The model under review builds one solid part; all positions refer to its coordinate system, in mm. A direction names the side the tool comes from. Coordinates: 2 decimals unless noted, no trailing zeros. Order: outer loops, then holes, each group sorted by start corner. A loop starts at its lowest first (then second) coordinate and runs counter-clockwise, first axis right, second up. Notation, with made-up numbers: M 56.5,84.25 L 68.5,84.25 A21 cw 68.5,101.25 Z; hole C 47,71 d6. An arc over 180 degrees is marked long. One line per item, written item: value.
```python
from build123d import *

# Parameters (mm, degrees)
F0_W         = 5
F0_H         = 5
F1_DEPTH     = 5
F2_DEPTH     = 15
F2_TAPER     = 5
F4_DEPTH     = 2.5
F5_T4_DEPTH  = 8.4
F5_T9_DEPTH  = 8.4
F5_T14_DEPTH = 8.4
F5_T19_DEPTH = 8.4
F5_T24_DEPTH = 8.4
F5_T29_DEPTH = 8.4
F5_T34_DEPTH = 8.4
F5_T39_DEPTH = 8.4
F6_T1_DEPTH  = 65.9153400942
F6_T6_DEPTH  = 63.5246599058
F6_T12_DEPTH = 63.5246599058


# Not quite as in the source:
# - a fillet or chamfer that OpenCascade refuses, or shapes differently, is made with other operations: its cross-section is extruded or revolved along the edge and cut away or added


with BuildPart() as f1:
    # F0 (on Top) → F1 (new body)
    with BuildSketch(Plane.XY):
        with Locations((-2.5, 2.5)):
            Rectangle(F0_W, F0_H)
    extrude(amount=F1_DEPTH)

    # F0 (on Top) → F2 (join)
    with BuildSketch(Plane.XY):
        with Locations((-2.5, 2.5)):
            Rectangle(F0_W, F0_H)
    extrude(amount=F2_DEPTH, taper=F2_TAPER)



with BuildPart() as f1b:
    # F0 (on Top) → F1, piece 2 (new body)
    with BuildSketch(Plane.XY):
        with Locations((57.5, 2.5)):
            Rectangle(F0_W, F0_H)
    extrude(amount=F1_DEPTH)

    # F0 (on Top) → F2, piece 2 (join)
    with BuildSketch(Plane.XY):
        with Locations((57.5, 2.5)):
            Rectangle(F0_W, F0_H)
    extrude(amount=F2_DEPTH, taper=F2_TAPER)


with BuildPart() as f1_1:
    add(f1.part)

    add(f1b.part)  # F4 merges F1b
    # F3 (on face) → F4 (join)
    with BuildSketch(Plane.XY.offset(15)):
        Polygon((-1.3123299529, 3.6876700471), (-3.6876700471, 3.6876700471), (-3.6876700471, 1.3123299529), (-1.3123299529, 1.3123299529), (56.3123299529, 1.3123299529), (58.6876700471, 1.3123299529), (58.6876700471, 3.6876700471), (56.3123299529, 3.6876700471), align=None)
    extrude(amount=F4_DEPTH)

    # F5: fillet of radius 1.18 on 4 edges, made by hand


with BuildPart() as f5_tool2:
    # F5_s3 → F5_t4 (new body)
    with BuildSketch(Plane.XY.offset(12.05)):
        with BuildLine():
            ThreePointArc((58.6876700471, 2.5076700471), (58.3420560489, 3.3420560489), (57.5076700471, 3.6876700471))
            Line((57.5076700471, 3.6876700471), (58.6876700471, 3.6876700471))
            Line((58.6876700471, 3.6876700471), (58.6876700471, 2.5076700471))
        make_face()
    extrude(amount=F5_T4_DEPTH)

    split(bisect_by=Plane(origin=(0, 4.9620193825, 0.4341204442), x_dir=(1, 0, 0), z_dir=(0, 0.9961946981, 0.0871557427)), keep=Keep.TOP)


with BuildPart() as f1_2:
    add(f1_1.part)

    # F5_t1: cut F5_tool2
    add(f5_tool2.part, mode=Mode.SUBTRACT)


with BuildPart() as f5_tool7:
    # F5_s8 → F5_t9 (new body)
    with BuildSketch(Plane.XY.offset(12.05)):
        with BuildLine():
            ThreePointArc((58.6876700471, 2.5076700471), (58.3420560489, 3.3420560489), (57.5076700471, 3.6876700471))
            Line((57.5076700471, 3.6876700471), (58.6876700471, 3.6876700471))
            Line((58.6876700471, 3.6876700471), (58.6876700471, 2.5076700471))
        make_face()
    extrude(amount=F5_T9_DEPTH)

    split(bisect_by=Plane(origin=(59.5442325904, 0, 5.20944533), x_dir=(0, 1, 0), z_dir=(0.9961946981, 0, 0.0871557427)), keep=Keep.TOP)


with BuildPart() as f1_3:
    add(f1_2.part)

    # F5_t6: cut F5_tool7
    add(f5_tool7.part, mode=Mode.SUBTRACT)


with BuildPart() as f5_tool12:
    # F5_s13 → F5_t14 (new body)
    with BuildSketch(Plane.XY.offset(12.05)):
        with BuildLine():
            ThreePointArc((57.5076700471, 1.3123299529), (58.3420560489, 1.6579439511), (58.6876700471, 2.4923299529))
            Line((58.6876700471, 2.4923299529), (58.6876700471, 1.3123299529))
            Line((58.6876700471, 1.3123299529), (57.5076700471, 1.3123299529))
        make_face()
    extrude(amount=F5_T14_DEPTH)

    split(bisect_by=Plane(origin=(59.5442325904, 0, 5.20944533), x_dir=(0, 1, 0), z_dir=(0.9961946981, 0, 0.0871557427)), keep=Keep.TOP)


with BuildPart() as f1_4:
    add(f1_3.part)

    # F5_t11: cut F5_tool12
    add(f5_tool12.part, mode=Mode.SUBTRACT)


with BuildPart() as f5_tool17:
    # F5_s18 → F5_t19 (new body)
    with BuildSketch(Plane.XY.offset(12.05)):
        with BuildLine():
            ThreePointArc((57.5076700471, 1.3123299529), (58.3420560489, 1.6579439511), (58.6876700471, 2.4923299529))
            Line((58.6876700471, 2.4923299529), (58.6876700471, 1.3123299529))
            Line((58.6876700471, 1.3123299529), (57.5076700471, 1.3123299529))
        make_face()
    extrude(amount=F5_T19_DEPTH)

    split(bisect_by=Plane(origin=(0, 0, 0), x_dir=(1, 0, 0), z_dir=(0, -0.9961946981, 0.0871557427)), keep=Keep.TOP)


with BuildPart() as f1_5:
    add(f1_4.part)

    # F5_t16: cut F5_tool17
    add(f5_tool17.part, mode=Mode.SUBTRACT)


with BuildPart() as f5_tool22:
    # F5_s23 → F5_t24 (new body)
    with BuildSketch(Plane.XY.offset(12.05)):
        with BuildLine():
            ThreePointArc((-2.5076700471, 3.6876700471), (-3.3420560489, 3.3420560489), (-3.6876700471, 2.5076700471))
            Line((-3.6876700471, 2.5076700471), (-3.6876700471, 3.6876700471))
            Line((-3.6876700471, 3.6876700471), (-2.5076700471, 3.6876700471))
        make_face()
    extrude(amount=F5_T24_DEPTH)

    split(bisect_by=Plane(origin=(-4.9620193825, 0, 0.4341204442), x_dir=(0, 1, 0), z_dir=(-0.9961946981, 0, 0.0871557427)), keep=Keep.TOP)


with BuildPart() as f1_6:
    add(f1_5.part)

    # F5_t21: cut F5_tool22
    add(f5_tool22.part, mode=Mode.SUBTRACT)


with BuildPart() as f5_tool27:
    # F5_s28 → F5_t29 (new body)
    with BuildSketch(Plane.XY.offset(12.05)):
        with BuildLine():
            ThreePointArc((-2.5076700471, 3.6876700471), (-3.3420560489, 3.3420560489), (-3.6876700471, 2.5076700471))
            Line((-3.6876700471, 2.5076700471), (-3.6876700471, 3.6876700471))
            Line((-3.6876700471, 3.6876700471), (-2.5076700471, 3.6876700471))
        make_face()
    extrude(amount=F5_T29_DEPTH)

    split(bisect_by=Plane(origin=(0, 4.9620193825, 0.4341204442), x_dir=(1, 0, 0), z_dir=(0, 0.9961946981, 0.0871557427)), keep=Keep.TOP)


with BuildPart() as f1_7:
    add(f1_6.part)

    # F5_t26: cut F5_tool27
    add(f5_tool27.part, mode=Mode.SUBTRACT)


with BuildPart() as f5_tool32:
    # F5_s33 → F5_t34 (new body)
    with BuildSketch(Plane.XY.offset(12.05)):
        with BuildLine():
            ThreePointArc((-2.5076700471, 1.3123299529), (-3.3420560489, 1.6579439511), (-3.6876700471, 2.4923299529))
            Line((-3.6876700471, 2.4923299529), (-3.6876700471, 1.3123299529))
            Line((-3.6876700471, 1.3123299529), (-2.5076700471, 1.3123299529))
        make_face()
    extrude(amount=F5_T34_DEPTH)

    split(bisect_by=Plane(origin=(-4.9620193825, 0, 0.4341204442), x_dir=(0, 1, 0), z_dir=(-0.9961946981, 0, 0.0871557427)), keep=Keep.TOP)


with BuildPart() as f1_8:
    add(f1_7.part)

    # F5_t31: cut F5_tool32
    add(f5_tool32.part, mode=Mode.SUBTRACT)


with BuildPart() as f5_tool37:
    # F5_s38 → F5_t39 (new body)
    with BuildSketch(Plane.XY.offset(12.05)):
        with BuildLine():
            ThreePointArc((-2.5076700471, 1.3123299529), (-3.3420560489, 1.6579439511), (-3.6876700471, 2.4923299529))
            Line((-3.6876700471, 2.4923299529), (-3.6876700471, 1.3123299529))
            Line((-3.6876700471, 1.3123299529), (-2.5076700471, 1.3123299529))
        make_face()
    extrude(amount=F5_T39_DEPTH)

    split(bisect_by=Plane(origin=(0, 0, 0), x_dir=(1, 0, 0), z_dir=(0, -0.9961946981, 0.0871557427)), keep=Keep.TOP)


with BuildPart() as f1_9:
    add(f1_8.part)

    # F5_t36: cut F5_tool37
    add(f5_tool37.part, mode=Mode.SUBTRACT)

    # F6: fillet of radius 1.18 on 8 edges, made by hand

    # F6_s2 → F6_t1 (cut)
    with BuildSketch(Plane.YZ.offset(-5.4576700471)):
        with BuildLine():
            ThreePointArc((3.6876700471, 16.32), (3.3420560489, 17.1543860018), (2.5076700471, 17.5))
            Line((2.5076700471, 17.5), (3.6876700471, 17.5))
            Line((3.6876700471, 17.5), (3.6876700471, 16.32))
        make_face()
        with BuildLine():
            ThreePointArc((2.4923299529, 17.5), (1.6579439511, 17.1543860018), (1.3123299529, 16.32))
            Line((1.3123299529, 16.32), (1.3123299529, 17.5))
            Line((1.3123299529, 17.5), (2.4923299529, 17.5))
        make_face()
    extrude(amount=F6_T1_DEPTH, mode=Mode.SUBTRACT)


with BuildPart() as f6_tool4:
    # F6_s5 → F6_t6 (new body)
    with BuildSketch(Plane.YZ.offset(59.2623299529)):
        with BuildLine():
            ThreePointArc((2.5076700471, 15), (3.3420560489, 15.3456139982), (3.6876700471, 16.18))
            Line((3.6876700471, 16.18), (3.6876700471, 15))
            Line((3.6876700471, 15), (2.5076700471, 15))
        make_face()
    extrude(amount=-F6_T6_DEPTH)

    split(bisect_by=Plane(origin=(54.5822132078, 0, -4.7753248858), x_dir=(0, 1, 0), z_dir=(-0.9961946981, 0, 0.0871557427)), keep=Keep.TOP)

    split(bisect_by=Plane(origin=(0, 0, 0), x_dir=(0, 1, 0), z_dir=(0.9961946981, 0, 0.0871557427)), keep=Keep.TOP)


with BuildPart() as f1_10:
    add(f1_9.part)

    # F6_t3: cut F6_tool4
    add(f6_tool4.part, mode=Mode.SUBTRACT)


with BuildPart() as f6_tool10:
    # F6_s11 → F6_t12 (new body)
    with BuildSketch(Plane.YZ.offset(-4.2623299529)):
        with BuildLine():
            ThreePointArc((2.4923299529, 15), (1.6579439511, 15.3456139982), (1.3123299529, 16.18))
            Line((1.3123299529, 16.18), (1.3123299529, 15))
            Line((1.3123299529, 15), (2.4923299529, 15))
        make_face()
    extrude(amount=F6_T12_DEPTH)

    split(bisect_by=Plane(origin=(54.5822132078, 0, -4.7753248858), x_dir=(0, 1, 0), z_dir=(-0.9961946981, 0, 0.0871557427)), keep=Keep.TOP)

    split(bisect_by=Plane(origin=(0, 0, 0), x_dir=(0, 1, 0), z_dir=(0.9961946981, 0, 0.0871557427)), keep=Keep.TOP)


with BuildPart() as f1_11:
    add(f1_10.part)

    # F6_t9: cut F6_tool10
    add(f6_tool10.part, mode=Mode.SUBTRACT)


solid = f1_11.part
```
(1) We need section C-C, the plane z = 8.25. State the section outline as (x, y) points, plus the area to 3 significant figures.
Geometry results:
outline: M -4.28,0.72 L -0.72,0.72 L -0.72,4.28 L -4.28,4.28 Z; M 55.72,0.72 L 59.28,0.72 L 59.28,4.28 L 55.72,4.28 Z
area: 25.3 mm2
(2) Insertion check: pin 1 Ø3 at (x, y) = (36.5, 1) entering from -Z; pin 2 Ø1.5 at (y, z) = (2, 11.5) entering from -X; pin 3 Ø0.7 at (x, z) = (22.5, 15.5) entering from -Y. Each pin has a flat end and moves straight along its axis. Give the tip position at first contact, or say it passes through.
Geometry results:
pin 1: stops at z = 15
pin 2: stops at x = -4.06
pin 3: stops at y = 1.36
(3) Mouldability with a two-part tool opening along Z and no side actions: class faces 3 (the flat face through (57.5, 4.8, 5)), 4 (the flat face through (57, 3, 0)), 5 (the flat face through (-4.8, 2.5, 5)), 6 (the flat face through (-3, 5, 2)) as +Z half, -Z half, draft (parallel to the pull), parting line (faces both ways), or undercut.
Geometry results:
face 3: undercut
face 4: -Z half
face 5: undercut
face 6: draft
(4) For L1, parallel to X at y = 3.25, z = 2.75; L2, parallel to X at y = 3.6, z = 8.5; L3, parallel to Z at x = 52.5, y = 2.5, list the stretches that pass through material, from the lowest coordinate up.
Geometry results:
L1: x = -5 to 0, 55 to 60
L2: x = -4.26 to -0.74, 55.74 to 59.26
L3: z = 15 to 17.5
(5) Tool access review of faces 1 (the flat face through (55, 2, 2)), 2 (the cylindrical face through (27.063, 3.351, 17.145)): name each direction out of +Z, -Z, +X, -X, +Y, -Y from which nothing blocks a thin tool from reaching the whole face with its end or side.
Geometry results:
face 1: -Z, +Y, -Y
face 2: +Z, +X, -X, +Y
(6) We need section A-A, the plane z = 2.5. State the section outline as (x, y) points.
Geometry results:
outline: M -5,0 L 0,0 L 0,5 L -5,5 Z; M 55,0 L 60,0 L 60,5 L 55,5 Z
